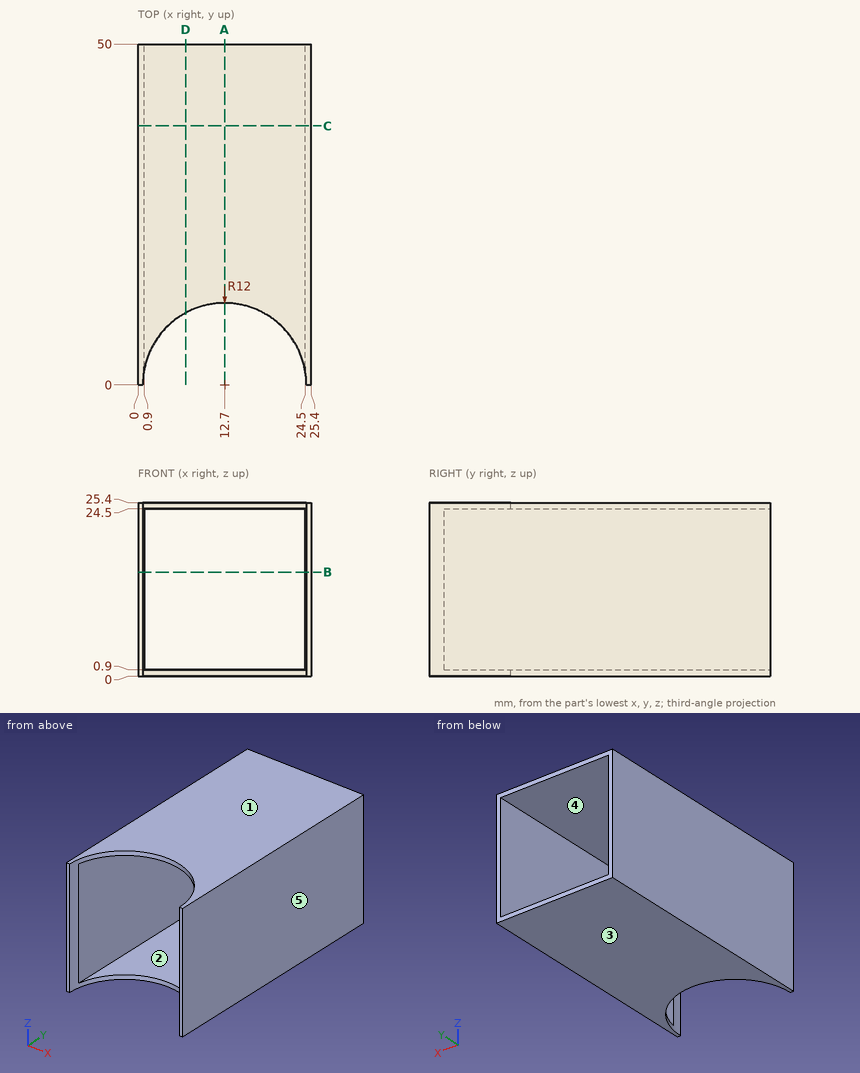
Check sheet for the drawn part. Datum: minimum x, y, z corner. Units: mm. A direction names the side the tool comes from. Give positions to 0.01 mm unless a question says otherwise; leave off trailing zeros. Order: outer loops, then holes, each group sorted by start corner. A loop starts at its lowest first (then second) coordinate and runs counter-clockwise, first axis right, second up. Notation, with made-up numbers: (71.25, -20) -> (99.25, -20) arc R17 cw to (99.25, 8) -> close; hole circle Ø11 at (40, -25.75). An arc over 180 degrees is marked (long way). Return JSON: item names as keys, results as strings.
1. Cross-section at A-A, the plane x = 12.7. Record the cut outline in (y, z).
From the geometry:
{"outline": "(12, 0) -> (50, 0) -> (50, 0.9) -> (12, 0.9) -> close; (12, 24.5) -> (50, 24.5) -> (50, 25.4) -> (12, 25.4) -> close"}
2. Set-up check for the marked faces 1 and 2: record each of +Z, -Z, +X, -X, +Y, -Y from which the full face is reachable in a straight line by a thin tool's end or side.
From the geometry:
{"face 1": "+Z, +X, -X, +Y, -Y", "face 2": "+Y, -Y"}
3. Material ranges on probe 1 along X at (y, z) = (46, 9.5), recorded low to high. Write a range as [from, to].
From the geometry:
{"probe 1": "[0, 0.9], [24.5, 25.4]"}
4. Mould release check, pull along Z, two halves, no side actions. Record for the marked faces 3, 4 and 5: +Z half, -Z half, draft (parallel to the pull), parting line (faces both ways), or undercut.
From the geometry:
{"face 3": "-Z half", "face 4": "undercut", "face 5": "draft"}
5. Cross-section at D-D, the plane x = 7. Record the cut outline in (y, z).
From the geometry:
{"outline": "(10.56, 0) -> (50, 0) -> (50, 0.9) -> (10.56, 0.9) -> close; (10.56, 24.5) -> (50, 24.5) -> (50, 25.4) -> (10.56, 25.4) -> close"}
6. Cross-section at C-C, the plane y = 38. Record the cut outline in (x, z).
From the geometry:
{"outline": "(0, 0) -> (25.4, 0) -> (25.4, 25.4) -> (0, 25.4) -> close; hole (0.9, 0.9) -> (24.5, 0.9) -> (24.5, 24.5) -> (0.9, 24.5) -> close"}
7. Go/stop test with flat-tipped pins: P1, Ø12, axis at y = 15, z = 15.5, coming from the -X side; P2, Ø8, axis at x = 15.5, z = 5.5, coming from the -Y side. Record where each tip stops, or that it passes through.
From the geometry:
{"P1": "x = 0", "P2": "through"}
8. Cross-section at B-B, the plane z = 15.25. Record the cut outline in (x, y).
From the geometry:
{"outline": "(0, 0) -> (0.7, 0) arc R12 cw to (0.9, 2.18) -> (0.9, 50) -> (0, 50) -> close; (24.5, 2.18) arc R12 cw to (24.7, 0) -> (25.4, 0) -> (25.4, 50) -> (24.5, 50) -> close"}
